from build123d import *

# Parameters (mm, degrees)
BOSS_EXTRUDE1_DEPTH = 8
SKETCH2_R           = 1.6
CUT_EXTRUDE1_DEPTH  = 9.5


with BuildPart() as part:
    # Sketch1 → Boss-Extrude1 (new body)
    with BuildSketch(Plane(origin=(0, 0, 0), x_dir=(0, 1, 0), z_dir=(0, 0, 1))):
        with BuildLine():
            Line((-16.649176641, -6.17541168), (-16.649176641, -5.37541168))
            Line((-16.649176641, -5.37541168), (-8.649176641, -5.37541168))
            Line((-8.649176641, -5.37541168), (-8.649176641, -4.37541168))
            Line((-8.649176641, -4.37541168), (-13.845329064, 4.62458832))
            ThreePointArc((-13.845329064, 4.62458832), (-13.552508741, 5.717408644), (-12.459688418, 5.42458832))
            Line((-12.459688418, 5.42458832), (-6.80165578, -4.37541168))
            Line((-6.80165578, -4.37541168), (-1.649176641, -4.37541168))
            Line((-1.649176641, -4.37541168), (-6.845329064, 4.62458832))
            ThreePointArc((-6.845329064, 4.62458832), (-6.552508741, 5.717408644), (-5.459688418, 5.42458832))
            Line((-5.459688418, 5.42458832), (0.19834422, -4.37541168))
            Line((0.19834422, -4.37541168), (0.503302498, -4.37541168))
            Line((0.503302498, -4.37541168), (6.161335136, 5.42458832))
            ThreePointArc((6.161335136, 5.42458832), (7.254155459, 5.717408644), (7.546975782, 4.62458832))
            Line((7.546975782, 4.62458832), (2.350823359, -4.37541168))
            Line((2.350823359, -4.37541168), (7.503302498, -4.37541168))
            Line((7.503302498, -4.37541168), (13.161335136, 5.42458832))
            ThreePointArc((13.161335136, 5.42458832), (14.254155459, 5.717408644), (14.546975782, 4.62458832))
            Line((14.546975782, 4.62458832), (9.350823359, -4.37541168))
            Line((9.350823359, -4.37541168), (9.350823359, -5.37541168))
            Line((9.350823359, -5.37541168), (17.350823359, -5.37541168))
            Line((17.350823359, -5.37541168), (17.350823359, -6.17541168))
            Line((17.350823359, -6.17541168), (-16.649176641, -6.17541168))
        make_face()
    extrude(amount=BOSS_EXTRUDE1_DEPTH)

    # Sketch2 → Cut-Extrude1 (cut)
    with BuildSketch(Plane(origin=(5.37541168, 0, 0), x_dir=(0, -1, 0), z_dir=(-1, 0, 0))):
        with Locations(Location((-13.350823359, 4, 0), (0, 0, 90))):
            Circle(SKETCH2_R)
        with Locations(Location((12.649176641, 4, 0), (0, 0, 90))):
            Circle(SKETCH2_R)
    extrude(amount=-CUT_EXTRUDE1_DEPTH, mode=Mode.SUBTRACT)


solid = part.part
Geometry: final body of the model. Coordinates: model frame, mm. A direction names the side the tool comes from. Coordinates: 2 decimals unless noted, no trailing zeros. Order: outer loops, then holes, each group sorted by start corner. A loop starts at its lowest first (then second) coordinate and runs counter-clockwise, first axis right, second up. Notation, with made-up numbers: M -7.5,55.25 L 42.5,55.25 A31 ccw 42.5,88.25 Z; hole C 57,-27.75 d9. An arc over 180 degrees is marked long. One line per question, with ' | ' between items. Start each with the question number.
Item 1: Cut plane D-D, the plane z = 1.75. Return the cut outline in (x, y), then the cut area to 3 significant figures.
Item 2: Set-up query: faces 4 (the flat face through (-0.188, 4.985, 3.944)), 5 (the flat face through (-0.456, 3.293, 3.944)), 6 (the flat face through (5.375, 11.5, 3.9)). Return all of +Z, -Z, +X, -X, +Y, -Y with unobstructed straight access to the full face (end or side cutting, diameter ignored); none if empty.
Item 3: Draft query along Z for faces 1 (the flat face through (4.375, 5, 4)), 2 (the flat face through (3, 2, 8)), 3 (the cylindrical face through (5.77, 11.93, 4.74)). Return one class per face: released by +Z, released by -Z, zero draft, split by the parting line, or undercut.
Item 4: Cut plane A-A, the plane z = 4. Count the separate pieces of the cut face and the enclosed holes in it, then the cut area to 3 significant figures.
Item 5: Cut plane B-B, the plane x = 1.75. Return the cut outline in (y, z).
Item 6: Cut plane C-C, the plane y = 11. Return the cut outline in (x, z).
Item 7: Ray query, probe 1 along Y at (x, z) = (5.7, 4); probe 2 along Y at (x, z) = (-3.5, 6.75); probe 3 along Y at (x, z) = (2.75, 7.25). Return the intervals inside material, ascending. Write a range as [from, to].
Item 8: Pin query (flat end, axial travel): pin 1 Ø3 at (x, z) = (0, 6) entering from -Y; pin 2 Ø1 at (x, z) = (2.5, 2) entering from +Y; pin 3 Ø2.5 at (y, z) = (12, 5) entering from -X. Return the tip coordinate at first contact, or that it passes through.
A:
1) outline: M -5.42,-12.46 A0.8 ccw -4.62,-13.85 L 4.38,-8.65 L 5.38,-8.65 L 5.38,-16.65 L 6.18,-16.65 L 6.18,17.35 L 5.38,17.35 L 5.38,9.35 L 4.38,9.35 L -4.62,14.55 A0.8 ccw -5.42,13.16 L 4.38,7.5 L 4.38,2.35 L -4.62,7.55 A0.8 ccw -5.42,6.16 L 4.38,0.5 L 4.38,0.2 L -5.42,-5.46 A0.8 ccw -4.62,-6.85 L 4.38,-1.65 L 4.38,-6.8 Z | area: 119 mm2
2) face 4: +Z, -Z | face 5: +Z, -Z, -X | face 6: +Z, -Z, +Y
3) face 1: zero draft | face 2: released by +Z | face 3: undercut
4) separate pieces: 3 | enclosed holes: 0 | area: 114 mm2
5) outline: M -10.16,0 L -8.32,0 L -8.32,8 L -10.16,8 Z; M -3.16,0 L -1.32,0 L -1.32,8 L -3.16,8 Z; M 2.02,0 L 3.87,0 L 3.87,8 L 2.02,8 Z; M 9.02,0 L 10.87,0 L 10.87,8 L 9.02,8 Z
6) outline: M -1.68,0 L 1.52,0 L 1.52,8 L -1.68,8 Z; M 5.38,0 L 6.18,0 L 6.18,8 L 5.38,8 Z
7) probe 1: y = [-16.65, -14.25], [-11.05, 11.75], [14.95, 17.35] | probe 2: y = [-13.2, -11.35], [-6.2, -4.35], [5.05, 6.9], [12.05, 13.9] | probe 3: y = [-9.59, -7.74], [-2.59, -0.74], [1.44, 3.29], [8.44, 10.29]
8) pin 1: stops at y = -12.04 | pin 2: stops at y = 10.72 | pin 3: stops at x = -5.55
